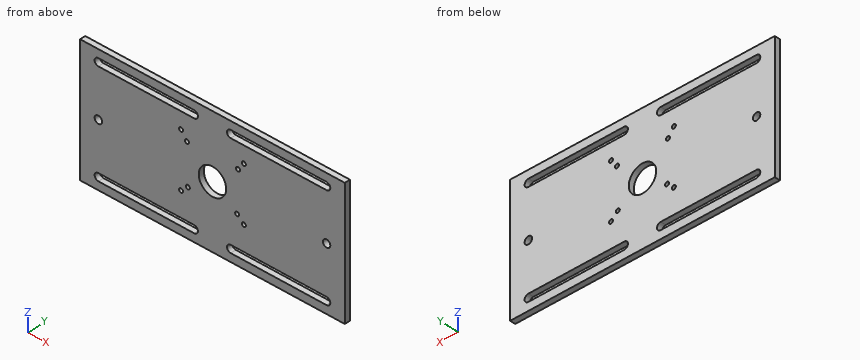
```python
from build123d import *

# Parameters (mm, degrees)
SKETCH_1_W      = 290
SKETCH_1_H      = 140
SKETCH_1_R      = 4.1
SKETCH_1_R_2    = 15
SKETCH_1_R_3    = 2.2
EXTRUDE_1_DEPTH = 6


with BuildPart() as part:
    # Эскиз1 → Бобышка-Вытянуть1 (new body)
    with BuildSketch(Plane(origin=(0, 0, 0), x_dir=(1, 0, 0), z_dir=(0, 1, 0))):
        Rectangle(SKETCH_1_W, SKETCH_1_H)
        with Locations((-125, 0)):
            Circle(SKETCH_1_R, mode=Mode.SUBTRACT)
        with Locations((125, 0)):
            Circle(SKETCH_1_R, mode=Mode.SUBTRACT)
        Circle(SKETCH_1_R_2, mode=Mode.SUBTRACT)
        with Locations((-34.4, 25.75)):
            Circle(SKETCH_1_R_3, mode=Mode.SUBTRACT)
        with Locations((34.4, 25.75)):
            Circle(SKETCH_1_R_3, mode=Mode.SUBTRACT)
        with Locations((-28, -26)):
            Circle(SKETCH_1_R_3, mode=Mode.SUBTRACT)
        with Locations((-34.4, -34.75)):
            Circle(SKETCH_1_R_3, mode=Mode.SUBTRACT)
        with Locations((-27, 18.75)):
            Circle(SKETCH_1_R_3, mode=Mode.SUBTRACT)
        with Locations((28, -26)):
            Circle(SKETCH_1_R_3, mode=Mode.SUBTRACT)
        with Locations((27, 18.75)):
            Circle(SKETCH_1_R_3, mode=Mode.SUBTRACT)
        with Locations((34.4, -34.75)):
            Circle(SKETCH_1_R_3, mode=Mode.SUBTRACT)
        with BuildLine():
            Line((-125, 61.1), (-20, 61.1))
            ThreePointArc((-20, 61.1), (-15.9, 57), (-20, 52.9))
            Line((-20, 52.9), (-125, 52.9))
            ThreePointArc((-125, 52.9), (-129.1, 57), (-125, 61.1))
        make_face(mode=Mode.SUBTRACT)
        with BuildLine():
            Line((-125, -52.9), (-20, -52.9))
            ThreePointArc((-20, -52.9), (-15.9, -57), (-20, -61.1))
            Line((-20, -61.1), (-125, -61.1))
            ThreePointArc((-125, -61.1), (-129.1, -57), (-125, -52.9))
        make_face(mode=Mode.SUBTRACT)
        with BuildLine():
            Line((125, -61.1), (20, -61.1))
            ThreePointArc((20, -61.1), (15.9, -57), (20, -52.9))
            Line((20, -52.9), (125, -52.9))
            ThreePointArc((125, -52.9), (129.1, -57), (125, -61.1))
        make_face(mode=Mode.SUBTRACT)
        with BuildLine():
            Line((125, 52.9), (20, 52.9))
            ThreePointArc((20, 52.9), (15.9, 57), (20, 61.1))
            Line((20, 61.1), (125, 61.1))
            ThreePointArc((125, 61.1), (129.1, 57), (125, 52.9))
        make_face(mode=Mode.SUBTRACT)
    extrude(amount=EXTRUDE_1_DEPTH)


solid = part.part
```
Verification items for the finished model (mm, model axes). Round coordinates to 2 decimals unless told otherwise and drop trailing zeros. Order: outer loops, then holes, each group sorted by start corner. A loop starts at its lowest first (then second) coordinate and runs counter-clockwise, first axis right, second up. Notation, with made-up numbers: (52, -18.5) - (75, -18.5) arc R29 ccw to (75, 5.5) - close; hole circle Ø9 at (56.25, 28). An arc over 180 degrees is marked (long way). Use CSV: the item, a comma, the result in double quotes. Start each with the question number.
1) Thickness scan on L1, parallel to X at y = 3, z = -57.5; L2, parallel to Z at x = -115, y = 0.65; L3, parallel to X at y = 2.55, z = -18.75. Record the ranges inside material, lowest first.
2) Go/stop test with a flat-tipped pin: P1, Ø7, axis at x = 34.4, z = 34.75, coming from the +Y side. Record where the tip stops, or that it passes through.
3) Section check A-A, the plane z = 57. Record the cut outline in (x, y), plus the area to 3 significant figures.
4) Section check B-B, the plane y = 2.4. State how many separate pieces and enclosed holes the cut face has, plus the area to 3 significant figures.
5) Section check C-C, the plane x = -71. Record the cut outline in (y, z).
6) Section check D-D, the plane z = 0. Record the cut outline in (x, y).
Answers:
1,L1,"x = -145 to -129.07, -15.93 to 15.93, 129.07 to 145"
1,L2,"z = -70 to -61.1, -52.9 to 52.9, 61.1 to 70"
1,L3,"x = -145 to -29.2, -24.8 to 24.8, 29.2 to 145"
2,P1,"stops at y = 6"
3,outline,"(-145, 0) - (-129.1, 0) - (-129.1, 6) - (-145, 6) - close; (-15.9, 0) - (15.9, 0) - (15.9, 6) - (-15.9, 6) - close; (129.1, 0) - (145, 0) - (145, 6) - (129.1, 6) - close"
3,area,"382 mm²"
4,separate pieces,"1"
4,enclosed holes,"15"
4,area,"36,000 mm²"
5,outline,"(0, -70) - (6, -70) - (6, -61.1) - (0, -61.1) - close; (0, -52.9) - (6, -52.9) - (6, 52.9) - (0, 52.9) - close; (0, 61.1) - (6, 61.1) - (6, 70) - (0, 70) - close"
6,outline,"(-145, 0) - (-129.1, 0) - (-129.1, 6) - (-145, 6) - close; (-120.9, 0) - (-15, 0) - (-15, 6) - (-120.9, 6) - close; (15, 0) - (120.9, 0) - (120.9, 6) - (15, 6) - close; (129.1, 0) - (145, 0) - (145, 6) - (129.1, 6) - close"
